Work out the finished part from the listing and answer in its coordinate system (mm). A direction names the side the tool comes from. Give positions to 0.01 mm unless a question says otherwise; leave off trailing zeros. Write each loop counter-clockwise with the first axis right and the second up, starting at its lowest first coordinate (ties: lowest second). Pieces come first, ordered by that corner, then holes. Notation, with made-up numbers: (85.5, 55) -> (133.5, 55) arc R23 cw to (133.5, 75) -> close; hole circle Ø2 at (85.25, 73). An arc over 180 degrees is marked (long way). Write item = value, one per line. Start each with the question number.
from build123d import *

# Parameters (mm, degrees)
BOSS_EXTRUDE1_DEPTH = 4.8641
SKETCH2_RX          = 0.5842
SKETCH2_RY          = 0.387956749
BOSS_EXTRUDE2_DEPTH = 0.7874
SKETCH4_RX          = 0.5842
SKETCH4_RY          = 0.387956749
BOSS_EXTRUDE3_DEPTH = 0.7874
BOSS_EXTRUDE5_DEPTH = 2.1336
BOSS_EXTRUDE6_DEPTH = 2.0574
SKETCH5_7_R         = 2.3114
BOSS_EXTRUDE7_DEPTH = 2.0701
SKETCH6_R           = 1.5
CUT_EXTRUDE1_DEPTH  = 10.7282


with BuildPart() as part:
    # Sketch1 → Boss-Extrude1 (new body, symmetric)
    with BuildSketch(Plane.XY):
        with BuildLine():
            Line((5.46, -14), (-5.46, -14))
            ThreePointArc((-5.46, -14), (-7.256051224, -13.256051224), (-8, -11.46))
            Line((-8, -11.46), (-8, 11.46))
            ThreePointArc((-8, 11.46), (-7.256051224, 13.256051224), (-5.46, 14))
            Line((-5.46, 14), (5.46, 14))
            ThreePointArc((5.46, 14), (7.256051224, 13.256051224), (8, 11.46))
            Line((8, 11.46), (8, -11.46))
            ThreePointArc((8, -11.46), (7.256051224, -13.256051224), (5.46, -14))
        make_face()
    extrude(amount=BOSS_EXTRUDE1_DEPTH, both=True)

    # Sketch2 → Boss-Extrude2 (add)
    with BuildSketch(Plane(origin=(3, 0, 0), x_dir=(0, 0, -1), z_dir=(1, 0, 0))):
        Polygon((-3.1, 14), (-3.1, 16.7), (-2.4, 16.7), (-2.4, 23.1), (2.4, 23.1), (2.4, 16.7), (3.1, 16.7), (3.1, 14), align=None)
        with Locations(Location((0, 19.925), (0, 0, -90))):
            Ellipse(SKETCH2_RX, SKETCH2_RY, mode=Mode.SUBTRACT)
    extrude(amount=-BOSS_EXTRUDE2_DEPTH)

    # Sketch4 → Boss-Extrude3 (add)
    with BuildSketch(Plane(origin=(-3, 0, 0), x_dir=(0, 0, -1), z_dir=(1, 0, 0))):
        Polygon((2.4, 16.7), (2.4, 23.1), (-2.4, 23.1), (-2.4, 16.7), (-3.1, 16.7), (-3.1, 14), (3.1, 14), (3.1, 16.7), align=None)
        with Locations(Location((0, 19.925), (0, 0, -90))):
            Ellipse(SKETCH4_RX, SKETCH4_RY, mode=Mode.SUBTRACT)
    extrude(amount=BOSS_EXTRUDE3_DEPTH)

    # Sketch5 → Boss-Extrude5 (add, symmetric)
    with BuildSketch(Plane.XY):
        Polygon((-8, 2.7732), (-10.29004586, 2.7732), (-12.680902195, -24.554412958), (-12.124228598, -24.603115587), (-9.778, 2.2144), (-8, 2.2144), align=None)
    extrude(amount=BOSS_EXTRUDE5_DEPTH, both=True)

    # Sketch5_6 → Boss-Extrude6 (add, symmetric)
    with BuildSketch(Plane.XY):
        with BuildLine():
            Line((-12.680902195, -24.554412958), (-12.326701257, -20.505877705))
            Line((-12.326701257, -20.505877705), (-15.151301123, -20.258757238))
            ThreePointArc((-15.151301123, -20.258757238), (-14.390077946, -21.092333666), (-14.114420252, -22.187013172))
            ThreePointArc((-14.114420252, -22.187013172), (-14.493232166, -23.454953726), (-15.505502062, -24.307292491))
            Line((-15.505502062, -24.307292491), (-12.680902195, -24.554412958))
        make_face()
    extrude(amount=BOSS_EXTRUDE6_DEPTH, both=True)

    # Sketch5_7 → Boss-Extrude7 (add, symmetric)
    with BuildSketch(Plane.XY):
        with Locations((-16.425820252, -22.187013172)):
            Circle(SKETCH5_7_R)
    extrude(amount=BOSS_EXTRUDE7_DEPTH, both=True)

    # Sketch6 → Cut-Extrude1 (cut, through all)
    with BuildSketch(Plane.XY.offset(4.8641)):
        with Locations((-5.25, 11)):
            Circle(SKETCH6_R)
        with Locations((5.25, -11)):
            Circle(SKETCH6_R)
    extrude(amount=-CUT_EXTRUDE1_DEPTH, mode=Mode.SUBTRACT)


solid = part.part
(1) A cutting plane is placed at D-D, the plane y = -11. Write down the section's boundary in (x, z).
(2) For faces 4 (the flat face through (0, -14, 0)), 5 (the flat face through (-9, 2.773, 0)), 6 (the flat face through (-11, -10, -2.134)), 7 (the cylindrical face through (-7.236, -13.276, 0.068)), determine the directions among +Z, -Z, +X, -X, +Y, -Y from which every point of the face is accessible in a straight line to the end or side of a thin tool.
(3) A cutting plane is placed at C-C, the plane z = -3.75. Write down the section's boundary in (x, y), then the cut area to 3 significant figures.
(4) A cutting plane is placed at A-A, the plane y = 15. Write down the section's boundary in (x, z).
(5) A cutting plane is placed at B-B, the plane x = -4.75. Write down the section's boundary in (y, z).
(6) Determine the mould class of faces 1 (the flat face through (-10.968, -11.382, 0.03)), 2 (the flat face through (-9, 2.214, 0)), 3 (the cylindrical face through (7.276, -13.236, 0.068)) for opening direction X: pulls with the +X half, pulls with the -X half, needs draft (parallel to the pull), parting line crosses it, or undercut.
(7) Each of these flat-tipped pins is pushed along its axis until it touches: pin 1 (2.5 mm diameter, centred on x = 5.25, y = -11, fed in from +Z); pin 2 (0.6 mm diameter, centred on x = 2.5, y = 20, fed in from +Z); pin 3 (3 mm diameter, centred on x = -1, z = -1, fed in from -Y); pin 4 (5 mm diameter, centred on y = -4.5, z = 1.5, fed in from -X). Where does it stop, or does it pass through?
(8) Find the intervals of material crossed by line 1 along Y through (x, z) = (5.25, 2.25); line 2 along Y through (x, z) = (-5.25, 2.5); line 3 along X through (y, z) = (-4, -2), in increasing order.
Results list:
q1.outline = (-11.5, -2.13) -> (-10.93, -2.13) -> (-10.93, 2.13) -> (-11.5, 2.13) -> close; (-8, -4.86) -> (3.75, -4.86) -> (3.75, 4.86) -> (-8, 4.86) -> close; (6.75, -4.86) -> (8, -4.86) -> (8, 4.86) -> (6.75, 4.86) -> close
q2.face_4 = +Z, -Z, +X, -Y
q2.face_5 = +Z, -Z, -X, +Y
q2.face_6 = -Z, -X, +Y, -Y
q2.face_7 = +Z, -Z, -Y
q3.outline = (-8, -11.46) arc R2.54 ccw to (-5.46, -14) -> (5.46, -14) arc R2.54 ccw to (8, -11.46) -> (8, 11.46) arc R2.54 ccw to (5.46, 14) -> (-5.46, 14) arc R2.54 ccw to (-8, 11.46) -> close; hole circle Ø3 at (-5.25, 11); hole circle Ø3 at (5.25, -11)
q3.area = 428 mm²
q4.outline = (-3, -3.1) -> (-2.21, -3.1) -> (-2.21, 3.1) -> (-3, 3.1) -> close; (2.21, -3.1) -> (3, -3.1) -> (3, 3.1) -> (2.21, 3.1) -> close
q5.outline = (-14, -4.86) -> (9.59, -4.86) -> (9.59, 4.86) -> (-14, 4.86) -> close; (12.41, -4.86) -> (14, -4.86) -> (14, 4.86) -> (12.41, 4.86) -> close
q6.face_1 = undercut
q6.face_2 = undercut
q6.face_3 = pulls with the +X half
q7.pin_1 = through
q7.pin_2 = 2.4
q7.pin_3 = -14
q7.pin_4 = -11.15
q8.line_1 = -14 to -12.5, -9.5 to 14
q8.line_2 = -14 to 9.5, 12.5 to 14
q8.line_3 = -10.88 to -10.32, -8 to 8
